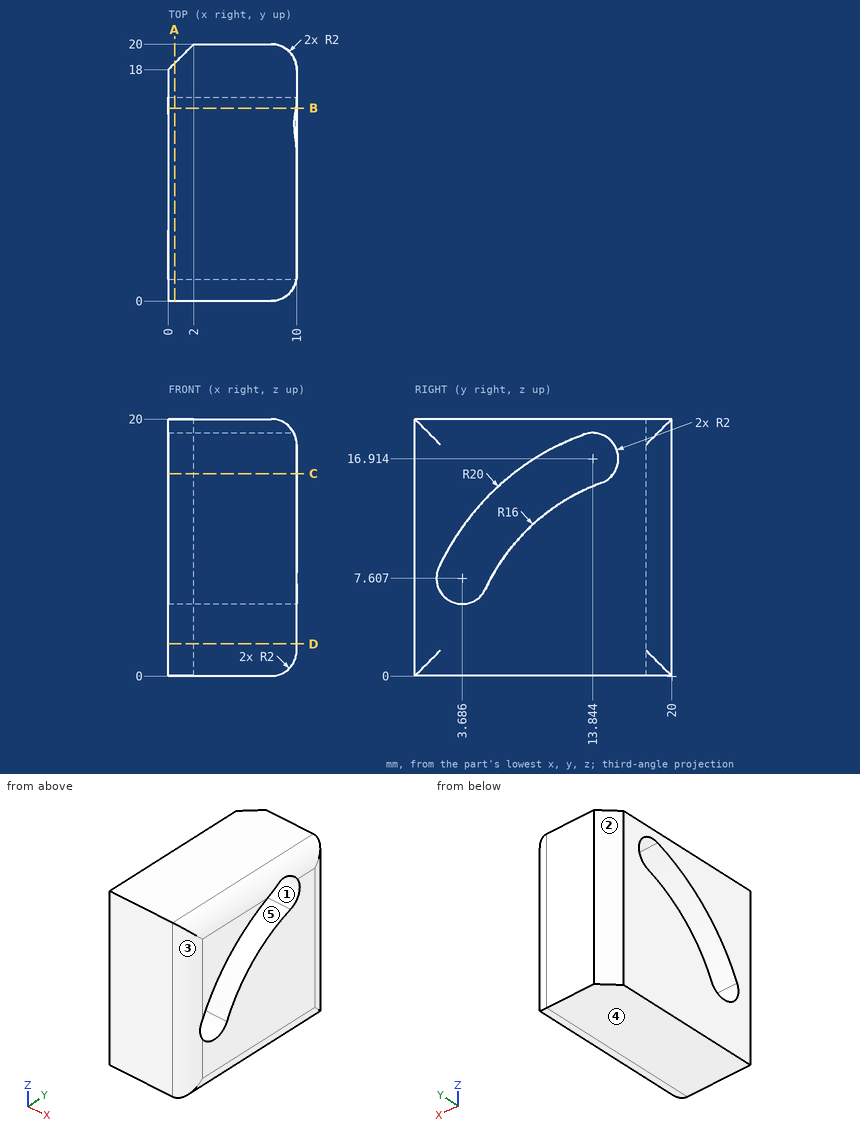
The drawing under review shows one solid part. Ordinate dimensions are in mm from its lowest x, y, z. A direction names the side the tool comes from. Round coordinates to 2 decimals unless told otherwise and drop trailing zeros. Loops run counter-clockwise (first coordinate to the right, second up) from the corner with the lowest first, then second, coordinate; pieces in that order, holes last. Notation, with made-up numbers: (86.5, 48) - (109.5, 48) arc R14 cw to (109.5, 58) - close; hole circle Ø10 at (-9.5, 1). An arc over 180 degrees is marked (long way). Use a Markdown table: item, result. Add a question column.
Q1. Add section D-D (z = 2.5). State the section outline as (x, y) points, plus the area to 3 significant figures.
Q2. Add section A-A (x = 0.5). State the section outline as (y, z) points (1 decimal).
Q3. Machinability: for the marked faces 4 and 5, which of the approach directions +Z, -Z, +X, -X, +Y, -Y give a long, thin tool a straight path to every point of the face, cutting with its end or side? Answer none if there is none.
Q4. Add section B-B (y = 15). State the section outline as (x, z) points, plus the area to 3 significant figures.
Q5. For probe 1 along Z at (x, y) = (9, 7.75) (1 decimal); probe 2 along Y at (x, z) = (2.5, 6.25) (1 decimal); probe 3 along Y at (x, z) = (2.5, 16.5) (1 decimal), list the stretches that pass through material, from the lowest coordinate up.
Q6. The part is to be moulded in two halves that separate along Y. For the marked faces 1, 2 and 3, say which applies: pulls with the +Y half, pulls with the -Y half, needs draft (parallel to the pull), parting line crosses it, or undercut.
Q7. Add section C-C (z = 15.75). State the section outline as (x, y) points.
Worked answers:
| question | item | result |
|---|---|---|
| 1 | outline | (0, 0) - (8, 0) arc R2 ccw to (10, 2) - (10, 18) arc R2 ccw to (8, 20) - (2, 20) - (0, 18) - close |
| 1 | area | 196 mm² |
| 2 | outline | (0, 0) - (18.5, 0) - (18.5, 20) - (0, 20) - close; hole (1.9, 8.5) arc R2 ccw to (5.5, 6.8) arc R16 cw to (14.5, 15) arc R2 ccw to (13.2, 18.8) arc R20 ccw to start |
| 3 | face 4 | -Z, +X, -X, +Y, -Y |
| 3 | face 5 | +X, -X |
| 4 | outline | (0, 0) - (8, 0) arc R2 ccw to (10, 2) - (10, 15.28) - (0, 15.28) - close; (0, 18.55) - (9.92, 18.55) arc R2 ccw to (8, 20) - (0, 20) - close |
| 4 | area | 166 mm² |
| 5 | probe 1 | 0.3 to 10.3, 15.8 to 19.7 |
| 5 | probe 2 | 0 to 2.2, 5.2 to 20 |
| 5 | probe 3 | 0 to 8.7, 15.8 to 20 |
| 6 | face 1 | undercut |
| 6 | face 2 | pulls with the +Y half |
| 6 | face 3 | pulls with the -Y half |
| 7 | outline | (0, 0) - (8, 0) arc R2 ccw to (10, 2) - (10, 7.67) - (0, 7.67) - close; (0, 15.47) - (10, 15.47) - (10, 18) arc R2 ccw to (8, 20) - (2, 20) - (0, 18) - close |
